from build123d import *

# Parameters (mm, degrees)
SKETCH1_R               = 38.1
BOSS_EXTRUDE1_DEPTH     = 16.66748
SKETCH2_R               = 19.84375
BOSS_EXTRUDE2_DEPTH     = 11.1125
CUT_EXTRUDE1_DEPTH      = 61.621343509
CUT_EXTRUDE2_DEPTH      = 11.1125
CUT_EXTRUDE2_DEPTH_BACK = 11.1125
SKETCH5_R               = 3.2639


with BuildPart() as part:
    # Sketch1 → Boss-Extrude1 (new body)
    with BuildSketch(Plane.XY):
        Circle(SKETCH1_R)
    extrude(amount=BOSS_EXTRUDE1_DEPTH)

    # Sketch2 → Boss-Extrude2 (add)
    with BuildSketch(Plane(origin=(0, 0, 0), x_dir=(-1, 0, 0), z_dir=(0, 0, -1))):
        with Locations(Location((0, 0, 0), (0, 0, 180))):
            Circle(SKETCH2_R)
    extrude(amount=BOSS_EXTRUDE2_DEPTH)

    # Sketch3 → Cut-Extrude1 (cut, through all)
    with BuildSketch(Plane(origin=(0, 0, -11.1125), x_dir=(-1, 0, 0), z_dir=(0, 0, -1))):
        with BuildLine():
            Line((-5.902263385, -1.078557803), (-8.315263385, -1.078557803))
            Line((-8.315263385, -1.078557803), (-8.315263385, 1.078557803))
            Line((-8.315263385, 1.078557803), (-5.902263385, 1.078557803))
            ThreePointArc((-5.902263385, 1.078557803), (6, 0), (-5.902263385, -1.078557803))
        make_face()
    extrude(amount=-CUT_EXTRUDE1_DEPTH, mode=Mode.SUBTRACT)

    # Sketch5 → Cut-Extrude2 (cut, two sides: drawn at the far end of the back side and taken through both)
    with BuildSketch(Plane(origin=(0, -9.525, 0), x_dir=(1, 0, 0), z_dir=(0, 1, 0)).offset(-CUT_EXTRUDE2_DEPTH_BACK)):
        with Locations(Location((0.599890424, 5.55752, 0), (0, 0, 90))):
            Circle(SKETCH5_R)
    extrude(amount=CUT_EXTRUDE2_DEPTH + CUT_EXTRUDE2_DEPTH_BACK, mode=Mode.SUBTRACT)

    # Sketch7 → Cut-Revolve1 (revolve, cut)
    with BuildSketch(Plane(origin=(0, 0, 0), x_dir=(0, 0, -1), z_dir=(1, 0, 0)), mode=Mode.PRIVATE) as cut_revolve1_sk:
        Polygon((-16.66748, 38.1), (0, 38.1), (-2.23774, 31.601131151), (-14.42974, 31.601131151), align=None)
    revolve(cut_revolve1_sk.sketch.rotate(Axis((0, 0, 16.66748), (0, 0, -1)), 90), axis=Axis((0, 0, 16.66748), (0, 0, -1)), mode=Mode.SUBTRACT)


solid = part.part
The model under review builds one solid part; all positions refer to its coordinate system, in mm. A direction names the side the tool comes from. Give positions to 0.01 mm unless a question says otherwise; leave off trailing zeros. Order: outer loops, then holes, each group sorted by start corner. A loop starts at its lowest first (then second) coordinate and runs counter-clockwise, first axis right, second up. Notation, with made-up numbers: M -9.5,69.25 L 36.5,69.25 A33 cw 36.5,104.25 Z; hole C 33,36.5 d7. An arc over 180 degrees is marked long. Answer in a Markdown table with one row per item. Add a question column.
1. Add section A-A on y = 0. State the section outline as (x, z) points, plus the area to 3 significant figures.
2. Add section B-B on z = 10.25. State the section outline as (x, y) points, plus the area to 3 significant figures.
3. For pin 1 Ø10 at (x, z) = (-3, 3) entering from +Y; pin 2 Ø1.1 at (y, z) = (0, 9) entering from -X; pin 3 Ø1.5 at (x, y) = (26.5, 26.5) entering from -Z, all flat-tipped, find the tip position at first contact; note any pin that passes through.
4. Add section C-C on z = -5.75. State the section outline as (x, y) points, plus the area to 3 significant figures.
5. Machinability: for faces 4 (the conical face through (-6.92, 31.16, 2.13)), 5 (the cylindrical face through (3.786, -12.326, -4.85)), 6 (the flat face through (7, -1.079, 3)), 7 (the flat face through (16, -16, 0)), 8 (the flat face through (4, -5, -11.112)), which of the approach directions +Z, -Z, +X, -X, +Y, -Y give a long, thin tool a straight path to every point of the face, cutting with its end or side? Answer none if there is none.
6. Mouldability with a two-part tool opening along Z and no side actions: class faces 1 (the cylindrical face through (30.142, -9.492, 8.419)), 2 (the flat face through (8.315, 0, 3)), 3 (the flat face through (-1, -8, 16.667)) as released by +Z, released by -Z, zero draft, split by the parting line, or undercut.
7. To check wall thickness, follow line 1 along Y through (x, z) = (0, 9); line 2 along Z through (x, y) = (-19, 8); line 3 along Y through (x, z) = (7, -6). State the ranges of each line that lie inside material, in increasing order.
The answers:
| question | item | result |
|---|---|---|
| 1 | outline | M -38.1,0 L -19.84,0 L -19.84,-11.11 L -6,-11.11 L -6,16.67 L -38.1,16.67 L -31.6,14.43 L -31.6,2.24 Z; M 8.32,-11.11 L 19.84,-11.11 L 19.84,0 L 38.1,0 L 31.6,2.24 L 31.6,14.43 L 38.1,16.67 L 8.32,16.67 Z |
| 1 | area | 1,130 mm2 |
| 2 | outline | C 0,0 d63.2; hole M 5.9,-1.08 L 8.32,-1.08 L 8.32,1.08 L 5.9,1.08 A6 ccw long Z |
| 2 | area | 3,020 mm2 |
| 3 | pin 1 | y = 38.1 |
| 3 | pin 2 | x = -31.6 |
| 3 | pin 3 | z = 0 |
| 4 | outline | M -2.66,-19.66 L -2.66,-5.38 A6 cw long 5.9,1.08 L 8.32,1.08 L 8.32,-1.08 L 5.9,-1.08 A6 cw 3.86,-4.6 L 3.86,-19.47 A19.84 ccw long Z |
| 4 | area | 1,030 mm2 |
| 5 | face 4 | none |
| 5 | face 5 | -Y |
| 5 | face 6 | +Z, -Z |
| 5 | face 7 | -Z |
| 5 | face 8 | -Z, +X, -X, +Y, -Y |
| 6 | face 1 | undercut |
| 6 | face 2 | zero draft |
| 6 | face 3 | released by +Z |
| 7 | line 1 | -31.6 to -6, 6 to 31.6 |
| 7 | line 2 | 0 to 16.67 |
| 7 | line 3 | -18.57 to -1.08, 1.08 to 18.57 |
